Model file for the job. Use its own axes, mm. A direction names the side the tool comes from. Coordinates: 2 decimals unless noted, no trailing zeros. Write each loop counter-clockwise with the first axis right and the second up, starting at its lowest first coordinate (ties: lowest second). Pieces come first, ordered by that corner, then holes. Notation, with made-up numbers: (36.5, 32.25) - (65.5, 32.25) arc R23 ccw to (65.5, 52.25) - close; hole circle Ø5 at (85.5, 19). An arc over 180 degrees is marked (long way). Put each result on its own line as item: value. Start each with the question number.
1. Drill centre lines: L1, parallel to X at y = 0, z = 0.55; L2, parallel to Y at x = 0, z = 11.2; L3, parallel to Z at x = 8, y = 0.75. Where is each one in solid material? Low to high. Write a range as from..to.
2. Saw through at B-B, the plane z = 3. Write the cut outline in (x, y), plus the area to 3 significant figures.
3. Which spindle directions (+Z, -Z, +X, -X, +Y, -Y) get a long thin tool onto all of the face, cutting with end or side? Do faces 1 (the face through (-9.223, -6.312, 11.192)), 2 (the face through (0, -11, 10.668)), 3 (the face through (0, -9.779, 6)), 4 (the face through (-5, 5, 4.064)). Say none if no direction does.
4. Saw through at D-D, the plane z = 6.25. Write the cut outline in (x, y), plus the area to 3 significant figures.
5. Saw through at C-C, the plane x = 4.5. Write the cut outline in (y, z).
6. Saw through at A-A, the plane y = -8.25. Write the cut outline in (x, z), plus the area to 3 significant figures.
7. Drop flat-ended pins along their axis: P1, Ø0.6, axis at y = -11.5, z = 0.5, coming from the -X side; P2, Ø3.5, axis at x = -0.5, z = 6, coming from the -Y side; P3, Ø6, axis at x = 3, z = 6.5, coming from the +Y side; P4, Ø2, axis at x = 0, y = 0, coming from the +Z side. Give the stop position or say it passes through.
8. Pull direction Z, two halves, no side cores. Call faces 5 (the face through (-0.372, -1.674, 0.376)), 6 (the face through (0, -11, 0.762)), 7 (the face through (-9.733, 9.1, 2.455)), 8 (the face through (0, -3, 11.43)): released by +Z, released by -Z, zero draft, split by the parting line, or undercut.
```python
from build123d import *

# Parameters (mm, degrees)
SKETCH1_R               = 1.7145
BOSS_EXTRUDE1_DEPTH     = 11.43
SKETCH2_W               = 9.906
SKETCH2_H               = 2.54
CUT_EXTRUDE1_DEPTH      = 21.259585188
CUT_EXTRUDE1_DEPTH_BACK = 21.259585188
SKETCH4_W               = 9.906
SKETCH4_H               = 20.955
SKETCH4_H_2             = 0.635
SKETCH3_R               = 5.588
BOSS_EXTRUDE2_DEPTH     = 4.064


with BuildPart() as part:
    # Sketch1 → Boss-Extrude1 (new body)
    with BuildSketch(Plane.XY):
        with BuildLine():
            Line((-2.286, 12.234260092), (-2.286, 10.939706577))
            ThreePointArc((-2.286, 10.939706577), (-11.176, 0), (-2.286, -10.939706577))
            Line((-2.286, -10.939706577), (-2.286, -12.234260092))
            ThreePointArc((-2.286, -12.234260092), (0, -12.446), (2.286, -12.234260092))
            Line((2.286, -12.234260092), (2.286, -10.939706577))
            ThreePointArc((2.286, -10.939706577), (11.176, 0), (2.286, 10.939706577))
            Line((2.286, 10.939706577), (2.286, 12.234260092))
            ThreePointArc((2.286, 12.234260092), (0, 12.446), (-2.286, 12.234260092))
        make_face()
        Circle(SKETCH1_R, mode=Mode.SUBTRACT)
    extrude(amount=BOSS_EXTRUDE1_DEPTH)

    # Sketch2 → Cut-Revolve1 (revolve, cut)
    with BuildSketch(Plane(origin=(0, 0, 0), x_dir=(0, 0, -1), z_dir=(1, 0, 0)), mode=Mode.PRIVATE) as cut_revolve1_sk:
        with Locations((-5.715, 12.446)):
            Rectangle(SKETCH2_W, SKETCH2_H)
    revolve(cut_revolve1_sk.sketch.rotate(Axis((0, 0, 11.43), (0, 0, -1)), 348.19710831), axis=Axis((0, 0, 11.43), (0, 0, -1)), mode=Mode.SUBTRACT)

    # Sketch4 → Cut-Extrude1 (cut, two sides: drawn at the far end of the back side and taken through both)
    with BuildSketch(Plane(origin=(0, 0, 0), x_dir=(0, 0, -1), z_dir=(1, 0, 0)).offset(-CUT_EXTRUDE1_DEPTH_BACK)):
        with Locations((-5.715, 0.6985)):
            Rectangle(SKETCH4_W, SKETCH4_H)
        with Locations((-5.715, -10.8585)):
            Rectangle(SKETCH4_W, SKETCH4_H_2)
    extrude(amount=CUT_EXTRUDE1_DEPTH + CUT_EXTRUDE1_DEPTH_BACK, mode=Mode.SUBTRACT)

    # Sketch3 → Boss-Extrude2 (add)
    with BuildSketch(Plane.XY):
        with Locations(Location((-5.477956234, 5.477956234, 0), (0, 0, 202.121055782))):
            Circle(SKETCH3_R)
    extrude(amount=BOSS_EXTRUDE2_DEPTH)


solid = part.part
```
Final values:
1. L1: x = -11.18..-1.71, 1.71..11.18
1. L2: y = -12.45..-1.71, 1.71..12.45
1. L3: z = 0..0.76, 10.67..11.43
2. outline: circle Ø11.18 at (-5.48, 5.48); (-5.41, -9.78) arc R11.18 ccw to (-3.71, -10.54) - (3.71, -10.54) arc R11.18 ccw to (5.41, -9.78) - close
2. area: 105 mm²
3. face 1: +Z, -X
3. face 2: +X, -X, -Y
3. face 3: +X, -X
3. face 4: +X, -X, +Y
4. outline: (-5.41, -9.78) arc R11.18 ccw to (-3.71, -10.54) - (3.71, -10.54) arc R11.18 ccw to (5.41, -9.78) - close
4. area: 7.05 mm²
5. outline: (-10.23, 0) - (10.23, 0) - (10.23, 0.76) - (-9.78, 0.76) - (-9.78, 10.67) - (10.23, 10.67) - (10.23, 11.43) - (-10.23, 11.43) - close
6. outline: (-7.54, 0) - (7.54, 0) - (7.54, 0.76) - (-7.54, 0.76) - close; (-7.54, 10.67) - (7.54, 10.67) - (7.54, 11.43) - (-7.54, 11.43) - close
6. area: 23.0 mm²
7. P1: stops at x = -2.29
7. P2: stops at y = -10.54
7. P3: stops at y = -9.78
7. P4: passes through
8. face 5: zero draft
8. face 6: undercut
8. face 7: undercut
8. face 8: released by +Z
